Autodesk Inventor part; units mm, degrees
ref_plane "YZ Plane" through (0, 0, 0) normal (1, 0, 0) x (0, 1, 0)
ref_plane "XZ Plane" through (0, 0, 0) normal (0, 1, 0) x (-1, 0, 0)
ref_plane "XY Plane" through (0, 0, 0) normal (0, 0, 1) x (1, 0, 0)
sketch "Sketch1" plane through (0, 0, 0) normal (0, 1, 0) x (-1, 0, 0)
  line L0 (-4.6, 4.6) -> (4.6, 4.6)
  line L1 (4.6, 4.6) -> (4.6, -4.6)
  line L2 (4.6, -4.6) -> (-4.6, -4.6)
  line L3 (-4.6, -4.6) -> (-4.6, 4.6)
  point P0 (0, 0)
  dimension "d0" = 9.2
  dimension "d1" = 9.2
  dimension "d2" = 4.6
  dimension "d3" = 4.6
extrude "Extrusion1" add sketch "Sketch1" along normal blind 4.5
sketch "Sketch3" plane through (0, 0, 0) normal (0, -1, 0) x (1, 0, 0)
  line L0 (-4.6, 4.6) -> (4.6, -4.6) construction
  line L1 (4.6, 4.6) -> (-4.6, -4.6) construction
  circle A0 centre (0, 0) radius 2.25
  point P0 (0, 0)
  point P1 (0, 0)
  dimension "d13" = 4.5
sketch "Sketch4" plane through (0, 4.5, 0) normal (0, 1, 0) x (1, 0, 0)
  circle A0 centre (0, 0) radius 1.3
  dimension "d10" = 2.6
extrude "Extrusion3" cut sketch "Sketch4" against normal blind 2
extrude "Extrusion4" cut sketch "Sketch3" against normal blind 2.5
equation "\"d0\" = 2 * BoltTrace"
equation "\"d1\" = d0"
equation "\"d4\" = ClassicThickness"
equation "\"d13\" = ServoHeadScrewTrace"
equation "\"d10\" = ServoScrewDiameterRequired"
equation "\"d11\" = MinimalThickness"
equation "\"d14\" = ServoHeadScrewThickness"
properties part number "ClassicScrewHeadTrace"
CAD build for the part. Positions are in the model's coordinates, mm. A direction names the side the tool comes from. Give positions to 0.01 mm unless a question says otherwise; leave off trailing zeros. Order: outer loops, then holes, each group sorted by start corner. A loop starts at its lowest first (then second) coordinate and runs counter-clockwise, first axis right, second up. Notation, with made-up numbers: (-20, 81) - (-1, 81) arc R28 ccw to (-1, 120) - close; hole circle Ø4 at (-29.75, 16.5). An arc over 180 degrees is marked (long way). Answer in a Markdown table with one row per item.
1. Tool access for faces 1 (the cylindrical face through (-0.29, 1.23, 2.23)), 2 (the flat face through (-4.6, 2, 0)): list every direction of +Z, -Z, +X, -X, +Y, -Y with a clear straight run to the whole face (end or side of a thin tool).
Data:
| item | result |
|---|---|
| face 1 | -Y |
| face 2 | +Z, -Z, -X, +Y, -Y |
2. Probe probe 1 along X at (y, z) = (4.1, 0); probe 2 along Z at (x, y) = (0, 1.5). List the from-to ranges inside material, lowest first. Write a range as [from, to].
Data:
| item | result |
|---|---|
| probe 1 | x = [-4.6, -1.3], [1.3, 4.6] |
| probe 2 | z = [-4.6, -2.25], [2.25, 4.6] |
3. Saw through at A-A, the plane x = 0. Give the cut face in (y, z), plus the area to 4 significant figures.
Data:
| item | result |
|---|---|
| outline | (0, -4.6) - (4.5, -4.6) - (4.5, -1.3) - (2.5, -1.3) - (2.5, -2.25) - (0, -2.25) - close; (0, 2.25) - (2.5, 2.25) - (2.5, 1.3) - (4.5, 1.3) - (4.5, 4.6) - (0, 4.6) - close |
| area | 24.95 mm² |
4. Saw through at B-B, the plane z = 0. Give the cut face in (x, y).
Data:
| item | result |
|---|---|
| outline | (-4.6, 0) - (-2.25, 0) - (-2.25, 2.5) - (-1.3, 2.5) - (-1.3, 4.5) - (-4.6, 4.5) - close; (1.3, 2.5) - (2.25, 2.5) - (2.25, 0) - (4.6, 0) - (4.6, 4.5) - (1.3, 4.5) - close |
5. Saw through at D-D, the plane x = 2. Give the cut face in (y, z).
Data:
| item | result |
|---|---|
| outline | (0, -4.6) - (4.5, -4.6) - (4.5, 4.6) - (0, 4.6) - (0, 1.03) - (2.5, 1.03) - (2.5, -1.03) - (0, -1.03) - close |
6. Saw through at C-C, the plane y = 4.15. Give the cut face in (x, z), plus the area to 3 significant figures.
Data:
| item | result |
|---|---|
| outline | (-4.6, -4.6) - (4.6, -4.6) - (4.6, 4.6) - (-4.6, 4.6) - close; hole circle Ø2.6 at (0, 0) |
| area | 79.3 mm² |
7. Pull direction Z, two halves, no side cores. Call faces 3 (the flat face through (1.1, 4.5, 1.1)), 4 (the flat face through (0, 2, 4.6)), 5 (the flat face through (0, 2, -4.6)), 6 (the flat face through (0, 2.5, -1.5)): pulls with the +Z half, pulls with the -Z half, needs draft (parallel to the pull), parting line crosses it, or undercut.
Data:
| item | result |
|---|---|
| face 3 | needs draft |
| face 4 | pulls with the +Z half |
| face 5 | pulls with the -Z half |
| face 6 | undercut |
